For this review, take the finished solid that the model builds, in its own axes (mm). A direction names the side the tool comes from. Round coordinates to 2 decimals unless told otherwise and drop trailing zeros. Order: outer loops, then holes, each group sorted by start corner. A loop starts at its lowest first (then second) coordinate and runs counter-clockwise, first axis right, second up. Notation, with made-up numbers: (-17.75, -22) -> (29.25, -22) arc R30 cw to (29.25, 17) -> close; hole circle Ø11 at (88, 56). An arc over 180 degrees is marked (long way). Use a Markdown table: item, result. Add a question column.
1) Wall thickness on line 1 along Y through (x, z) = (45, -112); line 2 along X through (y, z) = (719.5, -535); line 3 along Z through (x, y) = (-131.5, 900.5): over which ranges is each line inside the solid? List them lowest first. Write a range as [from, to].
2) Consider section D-D (x = 1087.5). State the section outline as (y, z) points, plus the area to 3 significant figures.
3) Consider section B-B (z = -198.5). State the section outline as (x, y) points.
4) Consider section C-C (y = 508). State the section outline as (x, z) points.
5) Draft analysis for pull direction Y (two halves, no side actions). For faces 3 (the face through (914.4, 275, -341)), 4 (the face through (635, 548, -330)), 5 (the face through (1315.11, 630.89, -142.75)), state which applies: pulls with the +Y half, pulls with the -Y half, needs draft (parallel to the pull), parting line crosses it, or undercut.
6) Clearance check with flat-ended pins moving along their axes: P1, Ø10, axis at y = 303, z = -16.5, coming from the +X side; P2, Ø1.5, axis at y = 396.5, z = -176, coming from the -X side; P3, Ø1.5, axis at y = 225, z = -588.5, coming from the -X side. State where each tip first meets the part, or that it passes through.
7) Machinability: for faces 1 (the face through (237, 779.639, -330)), 2 (the face through (1727.2, 505, -332)), which of the approach directions +Z, -Z, +X, -X, +Y, -Y give a long, thin tool a straight path to every point of the face, cutting with its end or side? Answer none if there is none.
8) Consider section A-A (y = 870.5). State the section outline as (x, z) points.
```python
from build123d import *

# Parameters (mm, degrees)
F1_DEPTH = 1016
F2_W     = 406.4
F2_H     = 457.2
F2_W_2   = 635
F3_DEPTH = 812.801
F4_R     = 228.6
F5_DEPTH = 812.8


with BuildPart() as f1:
    # F0 (on Front) → F1 (new body)
    with BuildSketch(Plane.XZ):
        with BuildLine():
            Line((914.4, 70.892677), (0, 70.892677))
            Line((0, 70.892677), (0, -132.307323))
            ThreePointArc((0, -132.307323), (143.684098, -191.823225), (203.2, -335.507323))
            ThreePointArc((203.2, -335.507323), (143.684098, -479.191421), (0, -538.707323))
            Line((0, -538.707323), (0, -741.907323))
            Line((0, -741.907323), (914.4, -741.907323))
            Line((914.4, -741.907323), (914.4, 70.892677))
        make_face()
        with BuildLine():
            Line((0, -132.307323), (0, 70.892677))
            ThreePointArc((0, 70.892677), (-287.368196, -48.139127), (-406.4, -335.507323))
            ThreePointArc((-406.4, -335.507323), (-287.368196, -622.875519), (0, -741.907323))
            Line((0, -741.907323), (0, -538.707323))
            ThreePointArc((0, -538.707323), (-203.2, -335.507323), (0, -132.307323))
        make_face()
    extrude(amount=-F1_DEPTH)

    # F2 (on face) → F3 (cut, through all)
    with BuildSketch(Plane.XY.offset(70.892677)):
        with Locations((-203.2, 551.038588)):
            Rectangle(F2_W, F2_H)
        with Locations((317.5, 551.038588)):
            Rectangle(F2_W_2, F2_H)
    extrude(amount=-F3_DEPTH, mode=Mode.SUBTRACT)

    # F4 (on face) → F5 (join)
    with BuildSketch(Plane.YZ.offset(914.4)):
        with Locations((508, -335.507323)):
            Circle(F4_R)
    extrude(amount=F5_DEPTH)


solid = f1.part
```
Results list:
| question | item | result |
|---|---|---|
| 1 | line 1 | [0, 322.44], [779.64, 1016] |
| 1 | line 2 | [635, 914.4] |
| 1 | line 3 | [-720.04, -490.42], [-180.59, 49.03] |
| 2 | outline | circle Ø457.2 at (508, -335.51) |
| 2 | area | 164,000 mm2 |
| 3 | outline | (-382.61, 0) -> (-150.06, 0) -> (-150.06, 322.44) -> (-382.61, 322.44) -> close; (-382.61, 779.64) -> (-150.06, 779.64) -> (-150.06, 1016) -> (-382.61, 1016) -> close; (150.06, 0) -> (914.4, 0) -> (914.4, 325.01) -> (1727.2, 325.01) -> (1727.2, 690.99) -> (914.4, 690.99) -> (914.4, 1016) -> (150.06, 1016) -> (150.06, 779.64) -> (635, 779.64) -> (635, 322.44) -> (150.06, 322.44) -> close |
| 4 | outline | (635, -741.91) -> (914.4, -741.91) -> (914.4, -564.11) -> (1727.2, -564.11) -> (1727.2, -106.91) -> (914.4, -106.91) -> (914.4, 70.89) -> (635, 70.89) -> close |
| 5 | face 3 | needs draft |
| 5 | face 4 | undercut |
| 5 | face 5 | parting line crosses it |
| 6 | P1 | x = 914.4 |
| 6 | P2 | x = 635 |
| 6 | P3 | x = -318.64 |
| 7 | face 1 | +Z, -Z, -X |
| 7 | face 2 | +Z, -Z, +X, +Y, -Y |
| 8 | outline | (0, -741.91) -> (914.4, -741.91) -> (914.4, 70.89) -> (0, 70.89) arc R406.4 ccw to start; hole circle Ø406.4 at (0, -335.51) |
